```python
from build123d import *


with BuildPart() as part:
    # Esquisse1 → Révolution1 (revolve)
    with BuildSketch(Plane.XY, mode=Mode.PRIVATE) as r_volution1_sk:
        with BuildLine():
            Line((0, 0), (48.706777749, 0))
            Line((48.706777749, 0), (46.062888871, 4.579349866))
            Line((46.062888871, 4.579349866), (41.039040874, 4.579349866))
            ThreePointArc((41.039040874, 4.579349866), (37.503506968, 6.04381596), (36.039040874, 9.579349866))
            Line((36.039040874, 9.579349866), (36.039040874, 15))
            ThreePointArc((36.039040874, 15), (34.57457478, 18.535533906), (31.039040874, 20))
            Line((31.039040874, 20), (10, 20))
            Line((10, 20), (10, 10))
            Line((10, 10), (0, 10))
            Line((0, 10), (0, 0))
        make_face()
    revolve(r_volution1_sk.sketch.rotate(Axis((0, 0, 0), (1, 0, 0)), 90), axis=Axis((0, 0, 0), (1, 0, 0)))


solid = part.part
```
Model file for the job. Use its own axes, mm. A direction names the side the tool comes from. Coordinates: 2 decimals unless noted, no trailing zeros. Loops run counter-clockwise (first coordinate to the right, second up) from the corner with the lowest first, then second, coordinate; pieces in that order, holes last. Notation, with made-up numbers: (49.25, 86) -> (72.25, 86) arc R11 cw to (72.25, 106) -> close; hole circle Ø6 at (-3.75, -22). An arc over 180 degrees is marked (long way). Answer as a JSON object with one key per item and string values.
Q1. Flat gauge pins, fed straight in: P1, Ø10, axis at x = 34, z = -0.5, coming from the -Y side; P2, Ø2, axis at x = 32, y = -8.5, coming from the -Z side; P3, Ø5, axis at y = -9, z = -14.5, coming from the -X side. Where does each tip first touch, or does it go through?
Report:
{"P1": "stops at y = -20", "P2": "stops at z = -18.47", "P3": "stops at x = 10"}
Q2. Cut at B-B (x = 5.5). List the corners of the cut face in (y, z), and give its area (3 significant figures).
Report:
{"outline": "circle Ø20 at (0, 0)", "area": "314 mm2"}
Q3. 3-axis set-ups, long thin cutter, end or side, ignore diameter. For faces 1 (the flat face through (0, 0, 0)), 2 (the cylindrical face through (5, 0, -10)), 3 (the flat face through (36.039, 10, 0)): which of +Z, -Z, +X, -X, +Y, -Y reach the whole face in a straight line?
Report:
{"face 1": "+Z, -Z, -X, +Y, -Y", "face 2": "-X", "face 3": "+X"}
Q4. Cut at A-A (x = 30). List the corners of the cut face in (y, z).
Report:
{"outline": "circle Ø40 at (0, 0)"}
Q5. Probe probe 1 along Z at (x, y) = (31, 0.5); probe 2 along X at (y, z) = (-10, 11); probe 3 along X at (y, z) = (0.5, 1.5). List the from-to ranges inside material, lowest first.
Report:
{"probe 1": "z = -19.99 to 19.99", "probe 2": "x = 10 to 36.04", "probe 3": "x = 0 to 47.79"}
